Read the model definition and answer for the solid it produces. Units are mm, in the model's axes. Give positions to 0.01 mm unless a question says otherwise; leave off trailing zeros. Order: outer loops, then holes, each group sorted by start corner. A loop starts at its lowest first (then second) coordinate and runs counter-clockwise, first axis right, second up. Notation, with made-up numbers: (-13, 32) -> (43, 32) arc R16 ccw to (43, 47) -> close; hole circle Ø9 at (22, 35.5). An arc over 180 degrees is marked (long way). Answer as CSV lines item,"result". Start each with the question number.
1) Find section C-C (z = 59). Determine the outline of the cut face in (x, y).
2) Find section A-A (y = 9). State how many separate pieces and enclosed holes the cut face has, and give its area (3 significant figures).
3) The mould has two halves that part along X. Classify faces 1 (the face through (80, 6, -46)), 2 (the face through (61.5, 7, -52)): +X half, -X half, draft (parallel to the pull), parting line (faces both ways), or undercut.
4) Find section D-D (z = -49). Determine the outline of the cut face in (x, y), and give its area (3 significant figures).
5) Flat-ended cylindrical pins translate along their axes: pin 1 Ø0.9 at (x, z) = (-84.5, -73) entering from -Y; pin 2 Ø5 at (x, z) = (85, -73) entering from -Y; pin 3 Ø9.5 at (x, z) = (59, -52.5) entering from -Y. Find the tip coordinate at first contact, or state that the pin passes through.
6) Find section B-B (x = -25). Determine the outline of the cut face in (y, z), and give its area (3 significant figures).
7) Straight lines are drawn through the part: L1, parallel to X at y = 4, z = -39; L2, parallel to Z at x = -38, y = 10. For each, find the intervals that lie inside material, in ascending order. Write a range as from..to.
```python
from build123d import *

# Parameters (mm, degrees)
SKETCH1_W           = 192
SKETCH1_H           = 192
SKETCH1_R           = 1.5
BOSS_EXTRUDE1_DEPTH = 13.85
SKETCH1_3_R         = 1.5
CUT_EXTRUDE1_DEPTH  = 11.85
SKETCH1_4_R         = 1.5
BOSS_EXTRUDE2_DEPTH = 3.5
CIRPATTERN1_COUNT   = 2
BOSS_EXTRUDE4_START = -2
SKETCH2_W           = 8.75
SKETCH2_H           = 27.8
SKETCH2_H_2         = 16
BOSS_EXTRUDE4_DEPTH = 9.5
BOSS_EXTRUDE5_START = -2
SKETCH2_3_R         = 3.5
BOSS_EXTRUDE5_DEPTH = 5.5


with BuildPart() as part:
    # Sketch1 → Boss-Extrude1 (new body)
    # profile 1 of 7: a face of its own
    with BuildSketch(Plane(origin=(0, 0, 0), x_dir=(1, 0, 0), z_dir=(0, 1, 0))):
        Rectangle(SKETCH1_W, SKETCH1_H)
        with Locations((62.5, -87.5)):
            Circle(SKETCH1_R, mode=Mode.SUBTRACT)
        with Locations((12, 85)):
            Circle(SKETCH1_R, mode=Mode.SUBTRACT)
        with Locations((85, 73)):
            Circle(SKETCH1_R, mode=Mode.SUBTRACT)
        with Locations((85, 0)):
            Circle(SKETCH1_R, mode=Mode.SUBTRACT)
        with Locations((85, -73)):
            Circle(SKETCH1_R, mode=Mode.SUBTRACT)
        with BuildLine():
            Line((5, 11.25), (65, 11.25))
            ThreePointArc((65, 11.25), (75.606601718, 15.643398282), (80, 26.25))
            Line((80, 26.25), (80, 65))
            ThreePointArc((80, 65), (75.606601718, 75.606601718), (65, 80))
            Line((65, 80), (-65, 80))
            ThreePointArc((-65, 80), (-75.606601718, 75.606601718), (-80, 65))
            Line((-80, 65), (-80, 26.25))
            ThreePointArc((-80, 26.25), (-75.606601718, 15.643398282), (-65, 11.25))
            Line((-65, 11.25), (-5, 11.25))
            ThreePointArc((-5, 11.25), (0, 16.25), (5, 11.25))
        make_face(mode=Mode.SUBTRACT)
    # profile 2 of 7: a face of its own
    with BuildSketch(Plane(origin=(0, 0, 0), x_dir=(1, 0, 0), z_dir=(0, 1, 0))):
        with BuildLine():
            ThreePointArc((5, 11.25), (0, 16.25), (-5, 11.25))
            Line((-5, 11.25), (-65, 11.25))
            ThreePointArc((-65, 11.25), (-75.606601718, 15.643398282), (-80, 26.25))
            Line((-80, 26.25), (-80, 65))
            ThreePointArc((-80, 65), (-75.606601718, 75.606601718), (-65, 80))
            Line((-65, 80), (65, 80))
            ThreePointArc((65, 80), (75.606601718, 75.606601718), (80, 65))
            Line((80, 65), (80, 26.25))
            ThreePointArc((80, 26.25), (75.606601718, 15.643398282), (65, 11.25))
            Line((65, 11.25), (5, 11.25))
        make_face()
    # profile 3 of 7: a face of its own
    with BuildSketch(Plane(origin=(0, 0, 0), x_dir=(1, 0, 0), z_dir=(0, 1, 0))):
        with Locations((62.5, -87.5)):
            Circle(SKETCH1_R)
    # profile 4 of 7: a face of its own
    with BuildSketch(Plane(origin=(0, 0, 0), x_dir=(1, 0, 0), z_dir=(0, 1, 0))):
        with Locations((85, -73)):
            Circle(SKETCH1_R)
    # profile 5 of 7: a face of its own
    with BuildSketch(Plane(origin=(0, 0, 0), x_dir=(1, 0, 0), z_dir=(0, 1, 0))):
        with Locations((85, 0)):
            Circle(SKETCH1_R)
    # profile 6 of 7: a face of its own
    with BuildSketch(Plane(origin=(0, 0, 0), x_dir=(1, 0, 0), z_dir=(0, 1, 0))):
        with Locations((85, 73)):
            Circle(SKETCH1_R)
    # profile 7 of 7: a face of its own
    with BuildSketch(Plane(origin=(0, 0, 0), x_dir=(1, 0, 0), z_dir=(0, 1, 0))):
        with Locations((12, 85)):
            Circle(SKETCH1_R)
    extrude(amount=BOSS_EXTRUDE1_DEPTH)

    # Sketch1<3> → Cut-Extrude1 (cut)
    with BuildSketch(Plane(origin=(0, 0, 0), x_dir=(1, 0, 0), z_dir=(0, 1, 0))):
        with BuildLine():
            ThreePointArc((5, 11.25), (0, 16.25), (-5, 11.25))
            Line((-5, 11.25), (-65, 11.25))
            ThreePointArc((-65, 11.25), (-75.606601718, 15.643398282), (-80, 26.25))
            Line((-80, 26.25), (-80, 65))
            ThreePointArc((-80, 65), (-75.606601718, 75.606601718), (-65, 80))
            Line((-65, 80), (65, 80))
            ThreePointArc((65, 80), (75.606601718, 75.606601718), (80, 65))
            Line((80, 65), (80, 26.25))
            ThreePointArc((80, 26.25), (75.606601718, 15.643398282), (65, 11.25))
            Line((65, 11.25), (5, 11.25))
        make_face()
        with Locations(Location((85, -73, 0), (0, 0, 270))):
            Circle(SKETCH1_3_R)
        with Locations(Location((85, 73, 0), (0, 0, 270))):
            Circle(SKETCH1_3_R)
        with Locations(Location((12, 85, 0), (0, 0, 270))):
            Circle(SKETCH1_3_R)
        with Locations(Location((85, 0, 0), (0, 0, 270))):
            Circle(SKETCH1_3_R)
    cut_extrude1 = extrude(amount=CUT_EXTRUDE1_DEPTH, mode=Mode.SUBTRACT)

    # Sketch1<4> → Boss-Extrude2 (add)
    with BuildSketch(Plane(origin=(0, 0, 0), x_dir=(1, 0, 0), z_dir=(0, 1, 0))):
        with Locations(Location((62.5, -87.5, 0), (0, 0, 270))):
            Circle(SKETCH1_4_R)
    boss_extrude2 = extrude(amount=-BOSS_EXTRUDE2_DEPTH)

    # CirPattern1: Cut-Extrude1, Boss-Extrude2 ×2 about axis
    cirpattern1_axis = Axis((0, 0, 0), (0, 1, 0))
    add([cut_extrude1.rotate(cirpattern1_axis, i * 360 / CIRPATTERN1_COUNT) for i in range(1, CIRPATTERN1_COUNT)], mode=Mode.SUBTRACT)
    add([boss_extrude2.rotate(cirpattern1_axis, i * 360 / CIRPATTERN1_COUNT) for i in range(1, CIRPATTERN1_COUNT)])

    # Sketch2 → Boss-Extrude4 (add)
    with BuildSketch(Plane(origin=(0, 13.85, 0), x_dir=(1, 0, 0), z_dir=(0, 1, 0)).offset(BOSS_EXTRUDE4_START)):
        with Locations((57.125, 52.1)):
            Rectangle(SKETCH2_W, SKETCH2_H)
        with Locations((-15.375, 48)):
            Rectangle(SKETCH2_W, SKETCH2_H_2)
        with Locations((-55.875, 52.1)):
            Rectangle(SKETCH2_W, SKETCH2_H)
    extrude(amount=-BOSS_EXTRUDE4_DEPTH)

    # Sketch2<3> → Boss-Extrude5 (add)
    with BuildSketch(Plane(origin=(0, 13.85, 0), x_dir=(1, 0, 0), z_dir=(0, 1, 0)).offset(BOSS_EXTRUDE5_START)):
        with Locations(Location((29, 49, 0), (0, 0, 270))):
            Circle(SKETCH2_3_R)
        with Locations(Location((-31, 49, 0), (0, 0, 270))):
            Circle(SKETCH2_3_R)
        with Locations(Location((29, -47, 0), (0, 0, 270))):
            Circle(SKETCH2_3_R)
        with Locations(Location((-31, -47, 0), (0, 0, 270))):
            Circle(SKETCH2_3_R)
    extrude(amount=-BOSS_EXTRUDE5_DEPTH)


solid = part.part
```
Findings below:
1,outline,"(-96, 0) -> (-80, 0) -> (-80, 11.85) -> (80, 11.85) -> (80, 0) -> (96, 0) -> (96, 13.85) -> (-96, 13.85) -> close"
2,separate pieces,"8"
2,enclosed holes,"10"
2,area,"16,100 mm²"
3,face 1,"undercut"
3,face 2,"undercut"
4,outline,"(-96, 0) -> (-80, 0) -> (-80, 11.85) -> (-60.25, 11.85) -> (-60.25, 2.35) -> (-51.5, 2.35) -> (-51.5, 11.85) -> (-34.5, 11.85) -> (-34.5, 6.35) -> (-27.5, 6.35) -> (-27.5, 11.85) -> (-19.75, 11.85) -> (-19.75, 2.35) -> (-11, 2.35) -> (-11, 11.85) -> (25.5, 11.85) -> (25.5, 6.35) -> (32.5, 6.35) -> (32.5, 11.85) -> (52.75, 11.85) -> (52.75, 2.35) -> (61.5, 2.35) -> (61.5, 11.85) -> (80, 11.85) -> (80, 0) -> (96, 0) -> (96, 13.85) -> (-96, 13.85) -> close"
4,area,"1,090 mm²"
5,pin 1,"y = 11.85"
5,pin 2,"y = 0"
5,pin 3,"y = 2.35"
6,outline,"(0, -96) -> (13.85, -96) -> (13.85, 96) -> (0, 96) -> (0, 80) -> (11.85, 80) -> (11.85, 11.25) -> (0, 11.25) -> (0, -11.25) -> (11.85, -11.25) -> (11.85, -80) -> (0, -80) -> close"
6,area,"1,030 mm²"
7,L1,"-96..-80, -60.25..-51.5, 52.75..61.5, 80..96"
7,L2,"-96..-80, -11.25..11.25, 80..96"
